Geometry: final body of the model. Coordinates: model frame, mm. A direction names the side the tool comes from. Coordinates: 2 decimals unless noted, no trailing zeros. Order: outer loops, then holes, each group sorted by start corner. A loop starts at its lowest first (then second) coordinate and runs counter-clockwise, first axis right, second up. Notation, with made-up numbers: (65, 45.5) -> (113, 45.5) arc R22 ccw to (113, 63.5) -> close; hole circle Ø7 at (53, -10). An arc over 180 degrees is marked (long way). Use CSV: the item, a comma, the result in double quotes. Start each with the question number.
from build123d import *

# Parameters (mm, degrees)
SKETCH_217_R        = 6
EXTRUDE_1_DEPTH     = 4
SKETCH_2_W          = 3.5
SKETCH_2_H          = 80
EXTRUDE_3_DEPTH     = 45
EXTRUDE_4_DEPTH     = 14.5
SKETCH_10_R         = 2.6
SKETCH_10_R_2       = 1.5
EXTRUDE_5_DEPTH     = 5
FILLET_1_R          = 2
FILLET_2_R          = 2
FILLET_3_R          = 10
FILLET_4_R          = 10
FILLET_5_R          = 5
SKETCH_12_R         = 1.5
CUT_EXTRUDE_1_DEPTH = 5


with BuildPart() as part:
    # Sketch 217 → 凸台-拉伸1 (new body)
    with BuildSketch(Plane(origin=(0, 0, 0), x_dir=(1, 0, 0), z_dir=(0, 1, 0))):
        with BuildLine():
            Line((79, 11.520697427), (79, 84.492095777))
            ThreePointArc((79, 84.492095777), (78.121320344, 86.613416121), (76, 87.492095777))
            Line((76, 87.492095777), (64.588699332, 87.492095777))
            ThreePointArc((64.588699332, 87.492095777), (0, 48.976277018), (-64.588699332, 87.492095777))
            Line((-64.588699332, 87.492095777), (-76, 87.492095777))
            ThreePointArc((-76, 87.492095777), (-78.121320344, 86.613416121), (-79, 84.492095777))
            Line((-79, 84.492095777), (-79, 11.520698809))
            ThreePointArc((-79, 11.520698809), (-78.121320344, 9.399378465), (-76, 8.520698809))
            Line((-76, 8.520698809), (76.002879086, 8.520698809))
            ThreePointArc((76.002879086, 8.520698809), (78.12233801, 9.400395239), (79, 11.520697427))
        make_face()
        with Locations(Location((68, 75.492095777, 0), (0, 0, 270))):  # turned: the seam where the file's is
            Circle(SKETCH_217_R, mode=Mode.SUBTRACT)
        with Locations(Location((-68, 75.492095777, 0), (0, 0, 270))):  # turned: the seam where the file's is
            Circle(SKETCH_217_R, mode=Mode.SUBTRACT)
    extrude(amount=EXTRUDE_1_DEPTH)

    # 草图2 → 凸台-拉伸3 (add, symmetric)
    with BuildSketch(Plane(origin=(0, 0, 0), x_dir=(0, 0, -1), z_dir=(1, 0, 0))):
        with Locations((10.270698809, -40)):
            Rectangle(SKETCH_2_W, SKETCH_2_H)
    extrude(amount=EXTRUDE_3_DEPTH, both=True)

    # 草图11 → 凸台-拉伸4 (add, symmetric)
    with BuildSketch(Plane(origin=(0, 0, 0), x_dir=(0, 0, -1), z_dir=(1, 0, 0))):
        Polygon((22.519495234, 0), (25.319495234, 0), (25.319495234, -13.290347232), (12.020698809, -28.288925016), (12.020698809, -25.13708489), (22.519495234, -13.2963882), align=None)
    extrude(amount=EXTRUDE_4_DEPTH, both=True)

    # 草图10 → 凸台-拉伸5 (add)
    with BuildSketch(Plane.XY.offset(-8.520698809)):
        with Locations(Location((23.511926173, -17.207974392, 0), (0, 0, 180))):  # turned: the seam where the file's is
            Circle(SKETCH_10_R)
        with Locations(Location((23.511926173, -17.207974392, 0), (0, 0, 180))):  # turned: the seam where the file's is
            Circle(SKETCH_10_R_2, mode=Mode.SUBTRACT)
        with Locations(Location((-24.77772075, -16.207974392, 0), (0, 0, 180))):  # turned: the seam where the file's is
            Circle(SKETCH_10_R)
        with Locations(Location((-24.77772075, -16.207974392, 0), (0, 0, 180))):  # turned: the seam where the file's is
            Circle(SKETCH_10_R_2, mode=Mode.SUBTRACT)
        with Locations(Location((8.524325101, -68.1489384, 0), (0, 0, 180))):  # turned: the seam where the file's is
            Circle(SKETCH_10_R)
        with Locations(Location((8.524325101, -68.1489384, 0), (0, 0, 180))):  # turned: the seam where the file's is
            Circle(SKETCH_10_R_2, mode=Mode.SUBTRACT)
    extrude(amount=EXTRUDE_5_DEPTH)

    # 圆角1
    fillet_1_edges = [part.edges().sort_by_distance(p)[0] for p in [
        (11.124325101, -68.1489384, -8.520698809),
    ]]
    fillet(fillet_1_edges, radius=FILLET_1_R)

    # 圆角2
    fillet_2_edges = [part.edges().sort_by_distance(p)[0] for p in [
        (26.111926173, -17.207974392, -8.520698809),
        (-22.17772075, -16.207974392, -8.520698809),
    ]]
    fillet(fillet_2_edges, radius=FILLET_2_R)

    # 圆角3
    fillet_3_edges = [part.edges().sort_by_distance(p)[0] for p in [
        (45, -80, -10.270698809),
    ]]
    fillet(fillet_3_edges, radius=FILLET_3_R)

    # 圆角4
    fillet_4_edges = [part.edges().sort_by_distance(p)[0] for p in [
        (-45, -80, -10.270698809),
    ]]
    fillet(fillet_4_edges, radius=FILLET_4_R)

    # 圆角5
    fillet_5_edges = [part.edges().sort_by_distance(p)[0] for p in [
        (0, 0, -25.319495234),
    ]]
    fillet(fillet_5_edges, radius=FILLET_5_R)

    # 草图12 → 切除-拉伸1 (cut)
    with BuildSketch(Plane.XY.offset(-8.520698809)):
        with Locations(Location((-24.77772075, -16.207974392, 0), (0, 0, 180))):  # turned: the seam where the file's is
            Circle(SKETCH_12_R)
        with Locations(Location((23.511926173, -17.207974392, 0), (0, 0, 180))):  # turned: the seam where the file's is
            Circle(SKETCH_12_R)
        with Locations(Location((8.524325101, -68.1489384, 0), (0, 0, 180))):  # turned: the seam where the file's is
            Circle(SKETCH_12_R)
    extrude(amount=-CUT_EXTRUDE_1_DEPTH, mode=Mode.SUBTRACT)


solid = part.part
(1) Section C-C (y = -45.5). Return loops of the section in (x, z), then the cut area to 3 significant figures.
(2) Line query: line 1 (Z direction, x = 26.5, y = -46.5); line 2 (Y direction, x = -71, z = -55); line 3 (Z direction, x = -5.5, y = -17.5). Output: solid intervals per line, ascending. Write a range as from..to.
(3) Section A-A (x = 68). Return loops of the section in (y, z).
(4) Mould query, pull axis X, two halves, no side actions, for faces 5 (the face through (7.127, -70.341, -5.042)), 6 (the face through (22.312, -14.901, -5.042)), 7 (the face through (41.99, -77.15, -10.3)). Classes: pulls with the +X half, pulls with the -X half, needs draft (parallel to the pull), parting line crosses it, or undercut.
(5) First-contact query: pin 1 (2.5 mm diameter, centred on x = -24.78, y = -16.21, fed in from -Z); pin 2 (14.5 mm diameter, centred on x = 4, y = -7.5, fed in from +Z); pin 3 (1.8 mm diameter, centred on y = -25.5, z = -11, fed in from -X); pin 4 (2 mm diameter, centred on x = -46, z = -39.5, fed in from -Y). Flat tips, straight axial feed; report the tip coordinate or a pass-through.
(6) Section D-D (x = 41). Return loops of the section in (y, z).
(7) Section B-B (y = -9). Return loops of the section in (x, z).
(8) Access query for faces 1 (the face through (-22.71, -14.63, -5.04)), 2 (the face through (0, -7, -22.519)), 3 (the face through (-14.5, -12, -23)), 4 (the face through (45, -35, -10)). Directions: +Z, -Z, +X, -X, +Y, -Y. A direction counts if a zero-diameter tool reaches every point of the face in a straight line with its end or side. Return the directions, or none.
Check sheet entries:
1,outline,"(-45, -12.02) -> (45, -12.02) -> (45, -8.52) -> (-45, -8.52) -> close"
1,area,"315 mm^2"
2,line 1,"z = -12.02..-8.52"
2,line 2,"y = 0..4"
2,line 3,"z = -21.59..-18.79, -12.02..-8.52"
3,outline,"(0, -87.49) -> (4, -87.49) -> (4, -81.49) -> (0, -81.49) -> close; (0, -69.49) -> (4, -69.49) -> (4, -8.52) -> (0, -8.52) -> close"
4,face 5,"parting line crosses it"
4,face 6,"undercut"
4,face 7,"pulls with the +X half"
5,pin 1,"passes through"
5,pin 2,"stops at z = -8.52"
5,pin 3,"stops at x = -45"
5,pin 4,"stops at y = 0"
6,outline,"(-78, -12.02) -> (0, -12.02) -> (0, -61.49) -> (4, -61.49) -> (4, -8.52) -> (-78, -8.52) -> close"
7,outline,"(-45, -12.02) -> (45, -12.02) -> (45, -8.52) -> (-45, -8.52) -> close; (-14.5, -25.32) -> (14.5, -25.32) -> (14.5, -22.52) -> (-14.5, -22.52) -> close"
8,face 1,"+Z"
8,face 2,"+X, -X"
8,face 3,"-Z, -X, -Y"
8,face 4,"+Z, -Z, +X, -Y"
